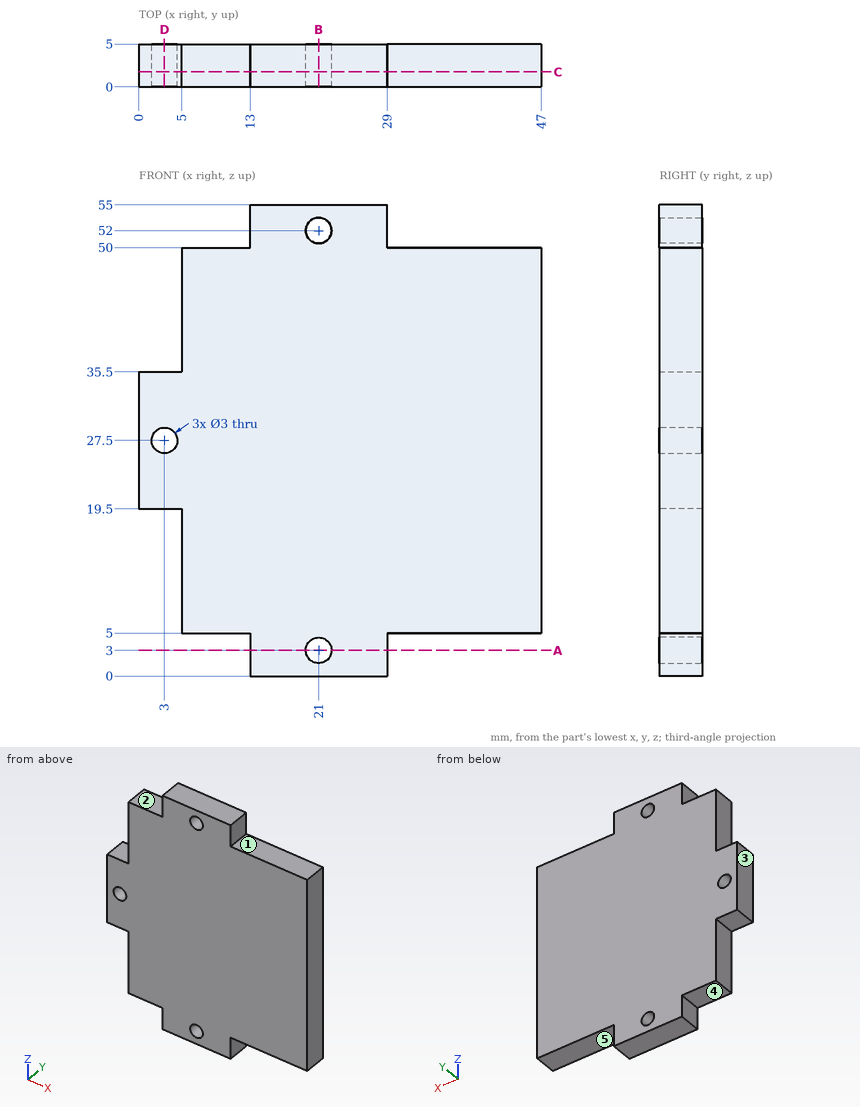
Could you check a few things on this drawing? It's one solid part, dimensions in mm from its lowest x, y, z. A direction names the side the tool comes from. Coordinates: 2 decimals unless noted, no trailing zeros. Write each loop counter-clockwise with the first axis right and the second up, starting at its lowest first coordinate (ties: lowest second). Pieces come first, ordered by that corner, then holes. Notation, with made-up numbers: (3.5, -18.5) - (22.5, -18.5) arc R35 cw to (22.5, 14.5) - close; hole circle Ø3 at (34, -15.75). An arc over 180 degrees is marked (long way). Put each result on its own line as item: value. Start each with the question number.
Q1. I want a section at A-A on z = 3. Write out the boundary of the cut face in (x, y).
Q2. Please list where these lines run through material, in increasing order: L1, parallel to X at y = 2.8, z = 3; L2, parallel to X at y = 2.95, z = 27.5; L3, parallel to X at y = 3.1, z = 45.
Q3. I'm going to push flat-ended pins straight in: P1, Ø2.5, axis at x = 21, z = 3, coming from the -Y side; P2, Ø2.5, axis at x = 3.5, y = 3.5, coming from the -Z side; P3, Ø2.5, axis at x = 36.5, y = 1.5, coming from the -Z side; P4, Ø1.5, axis at x = 8.5, y = 3, coming from the +Z side. Where does each tip first touch, or does it pass through?
Q4. I want a section at C-C on y = 1.75. Write out the boundary of the cut face in (x, z).
Q5. I want a section at D-D on x = 3. Write out the boundary of the cut face in (y, z).
Q6. Which directions (+Z, -Z, +X, -X, +Y, -Y) give clear straight access to the entire face, cutting with the end or side of a thin tool? Please do the marked faces 1, 2, 3, 4 and 5.
Q7. I want a section at B-B on x = 21. Write out the boundary of the cut face in (y, z), plus the area to 3 significant figures.
Checks:
1. outline: (13, 0) - (19.5, 0) - (19.5, 5) - (13, 5) - close; (22.5, 0) - (29, 0) - (29, 5) - (22.5, 5) - close
2. L1: 13 to 19.5, 22.5 to 29
2. L2: 0 to 1.5, 4.5 to 47
2. L3: 5 to 47
3. P1: through
3. P2: z = 19.5
3. P3: z = 5
3. P4: z = 50
4. outline: (0, 19.5) - (5, 19.5) - (5, 5) - (13, 5) - (13, 0) - (29, 0) - (29, 5) - (47, 5) - (47, 50) - (29, 50) - (29, 55) - (13, 55) - (13, 50) - (5, 50) - (5, 35.5) - (0, 35.5) - close; hole circle Ø3 at (3, 27.5); hole circle Ø3 at (21, 3); hole circle Ø3 at (21, 52)
5. outline: (0, 19.5) - (5, 19.5) - (5, 26) - (0, 26) - close; (0, 29) - (5, 29) - (5, 35.5) - (0, 35.5) - close
6. face 1: +Z, +X, +Y, -Y
6. face 2: +Z, -X, +Y, -Y
6. face 3: +Z, -Z, -X, +Y, -Y
6. face 4: -Z, -X, +Y, -Y
6. face 5: -Z, +X, +Y, -Y
7. outline: (0, 0) - (5, 0) - (5, 1.5) - (0, 1.5) - close; (0, 4.5) - (5, 4.5) - (5, 50.5) - (0, 50.5) - close; (0, 53.5) - (5, 53.5) - (5, 55) - (0, 55) - close
7. area: 245 mm²
